```python
from build123d import *

# Parameters (mm, degrees)
SKETCH_1_W          = 85
SKETCH_1_H          = 120
EXTRUDE_1_DEPTH     = 10
SKETCH_2_W          = 65
SKETCH_2_H          = 60
SKETCH_2_W_2        = 49
SKETCH_2_H_2        = 44
EXTRUDE_2_DEPTH     = 110
FILLET_1_R          = 5
FILLET_2_R          = 12
SKETCH_3_R          = 2.1
CUT_EXTRUDE_1_DEPTH = 159.823801743
FILLET_3_R          = 20


with BuildPart() as part:
    # 草图1 → 凸台-拉伸1 (new body)
    with BuildSketch(Plane(origin=(0, 0, 0), x_dir=(1, 0, 0), z_dir=(0, 1, 0))):
        Rectangle(SKETCH_1_W, SKETCH_1_H)
    extrude(amount=EXTRUDE_1_DEPTH)

    # 草图2 → 凸台-拉伸2 (add)
    with BuildSketch(Plane(origin=(0, 10, 0), x_dir=(1, 0, 0), z_dir=(0, 1, 0))):
        Rectangle(SKETCH_2_W, SKETCH_2_H)
        Rectangle(SKETCH_2_W_2, SKETCH_2_H_2, mode=Mode.SUBTRACT)
    extrude(amount=EXTRUDE_2_DEPTH)

    # 圆角1
    fillet_1_edges = [part.edges().sort_by_distance(p)[0] for p in [
        (0, 0, -60),
        (42.5, 0, 0),
        (0, 0, 60),
        (-42.5, 0, 0),
        (-42.5, 5, -60),
        (42.5, 5, -60),
        (42.5, 5, 60),
        (-42.5, 5, 60),
    ]]
    fillet(fillet_1_edges, radius=FILLET_1_R)

    # 圆角2
    # the kernel refuses this fillet: 12 mm, written as the material it takes off along each edge
    with BuildSketch(Plane(origin=(62.5, 120, 30), x_dir=(0, -1, 0), z_dir=(-1, 0, 0)), Plane(origin=(-62.5, 120, -30), x_dir=(0, -1, 0), z_dir=(1, 0, 0))) as fillet_2_piece_1:
        with BuildLine():
            CenterArc((FILLET_2_R, -FILLET_2_R), FILLET_2_R, 90, 90)
            Line((0, -FILLET_2_R), (0, 0))
            Line((0, 0), (FILLET_2_R, 0))
        make_face()
    extrude(amount=125, mode=Mode.SUBTRACT)

    # 草图3 → 切除-拉伸1 (cut, through all)
    with BuildSketch(Plane(origin=(42.5, 0, 0), x_dir=(0, 0, -1), z_dir=(1, 0, 0))):
        with Locations(Location((-15, 112, 0), (0, 0, 180))):
            Circle(SKETCH_3_R)
        with Locations(Location((15, 112, 0), (0, 0, 180))):
            Circle(SKETCH_3_R)
        with Locations(Location((15, 77, 0), (0, 0, 180))):
            Circle(SKETCH_3_R)
        with Locations(Location((-15, 77, 0), (0, 0, 180))):
            Circle(SKETCH_3_R)
    extrude(amount=-CUT_EXTRUDE_1_DEPTH, mode=Mode.SUBTRACT)

    # 圆角3
    fillet_3_edges = [part.edges().sort_by_distance(p)[0] for p in [
        (0, 10, 30),
        (0, 10, -30),
    ]]
    fillet(fillet_3_edges, radius=FILLET_3_R)


solid = part.part
```
Design review of the part built by this model. Coordinates are the model's own, in mm. A direction names the side the tool comes from. Round coordinates to 2 decimals unless told otherwise and drop trailing zeros. Order: outer loops, then holes, each group sorted by start corner. A loop starts at its lowest first (then second) coordinate and runs counter-clockwise, first axis right, second up. Notation, with made-up numbers: (-26.75, 45.25) - (-12.75, 45.25) arc R16 cw to (-12.75, 64.25) - close; hole circle Ø5 at (57, 61.5). An arc over 180 degrees is marked (long way). Return JSON: item names as keys, results as strings.
Q1. Consider section D-D on x = 10.5. Write out the cut boundary in (y, z), plus the area to 3 significant figures.
Computed values:
{"outline": "(0, -55) arc R5 ccw to (5, -60) - (10, -60) - (10, -50) arc R20 cw to (30, -30) - (108, -30) arc R12 ccw to (119.31, -22) - (10, -22) - (10, 22) - (119.31, 22) arc R12 ccw to (108, 30) - (30, 30) arc R20 cw to (10, 50) - (10, 60) - (5, 60) arc R5 ccw to (0, 55) - close", "area": "3,060 mm2"}
Q2. Consider section C-C on y = 38. Write out the cut boundary in (x, z).
Computed values:
{"outline": "(-32.5, -30) - (32.5, -30) - (32.5, 30) - (-32.5, 30) - close; hole (-24.5, -22) - (24.5, -22) - (24.5, 22) - (-24.5, 22) - close"}
Q3. Consider section A-A on y = 77. Write out the cut boundary in (x, z), plus the area to 3 significant figures.
Computed values:
{"outline": "(-32.5, -30) - (32.5, -30) - (32.5, -17.1) - (24.5, -17.1) - (24.5, -22) - (-24.5, -22) - (-24.5, -17.1) - (-32.5, -17.1) - close; (-32.5, -12.9) - (-24.5, -12.9) - (-24.5, 12.9) - (-32.5, 12.9) - close; (-32.5, 17.1) - (-24.5, 17.1) - (-24.5, 22) - (24.5, 22) - (24.5, 17.1) - (32.5, 17.1) - (32.5, 30) - (-32.5, 30) - close; (24.5, -12.9) - (32.5, -12.9) - (32.5, 12.9) - (24.5, 12.9) - close", "area": "1,610 mm2"}
Q4. Wall thickness on L1, parallel to Y at x = -29, z = 15; L2, parallel to Z at x = -28.25, y = 77; L3, parallel to X at y = 55.5, z = -11.5: over which ranges is each line inside the solid? List them lowest first. Write a range as [from, to].
Computed values:
{"L1": "y = [0, 74.9], [79.1, 109.9], [114.1, 120]", "L2": "z = [-30, -17.1], [-12.9, 12.9], [17.1, 30]", "L3": "x = [-32.5, -24.5], [24.5, 32.5]"}
Q5. Consider section B-B on z = 15. Give the number of separate pieces and of enclosed holes in the cut face, plus the area to 3 significant figures.
Computed values:
{"separate pieces": "5", "enclosed holes": "0", "area": "2,460 mm2"}
Q6. For pin 1 Ø6.5 at (y, z) = (112, 15) entering from -X; pin 2 Ø10 at (x, y) = (-26.5, 82) entering from +Z; pin 3 Ø5.5 at (y, z) = (77, 15) entering from +X, all flat-tipped, find the tip position at first contact; note any pin that passes through.
Computed values:
{"pin 1": "stops at x = -32.5", "pin 2": "stops at z = 30", "pin 3": "stops at x = 32.5"}
Q7. The part is to be moulded in two halves that separate along X. For faces 1 (the flat face through (0, 64, -22)), 2 (the flat face through (-42.5, 7, 1)), 3 (the flat face through (0, 68, -30)), say which applies: pulls with the +X half, pulls with the -X half, needs draft (parallel to the pull), parting line crosses it, or undercut.
Computed values:
{"face 1": "undercut", "face 2": "pulls with the -X half", "face 3": "needs draft"}
Q8. Machinability: for faces 4 (the flat face through (0, 68, 30)), 5 (the flat face through (37, 10, -1)), 6 (the flat face through (-32.5, 64, 1)), 7 (the flat face through (32.5, 64, 1)), which of the approach directions +Z, -Z, +X, -X, +Y, -Y give a long, thin tool a straight path to every point of the face, cutting with its end or side? Answer none if there is none.
Computed values:
{"face 4": "+Z, +X, -X, +Y", "face 5": "+Y", "face 6": "+Z, -Z, -X, +Y", "face 7": "+Z, -Z, +X, +Y"}
